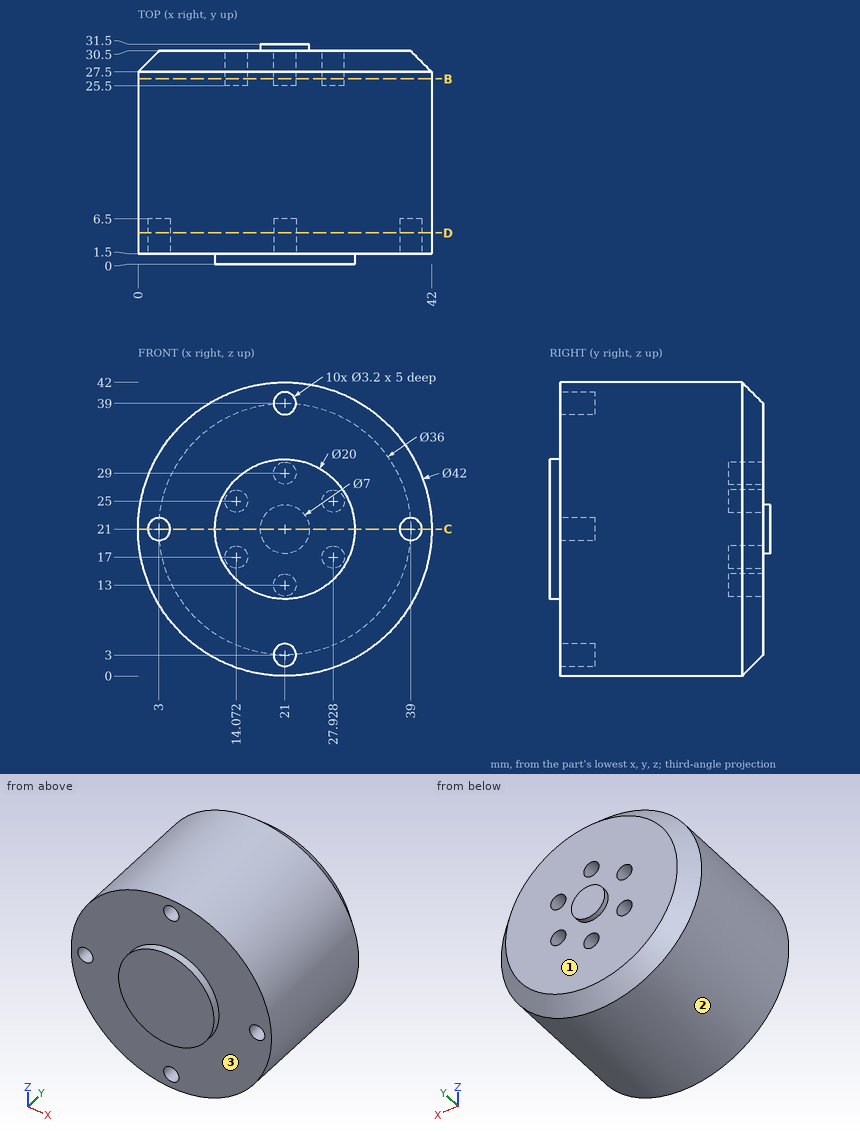
Study the drawing (mm; zero at the part's minimum x, y, z) and answer. Give positions to 0.01 mm unless a question says otherwise; leave off trailing zeros. Loops run counter-clockwise (first coordinate to the right, second up) from the corner with the lowest first, then second, coordinate; pieces in that order, holes last. Notation, with made-up numbers: M 20.25,49 L 48.25,49 A24 cw 48.25,63 Z; hole C 12.25,0 d7. An arc over 180 degrees is marked long. One line per item, written item: value.
1. Find the intervals of material crossed by probe 1 along X at (y, z) = (26, 25) (1 decimal); probe 2 along X at (y, z) = (28.3, 17); probe 3 along Z at (x, y) = (29, 27), in increasing order.
Found:
probe 1: 0.4 to 12.5, 15.7 to 26.3, 29.5 to 41.6
probe 2: 1.2 to 12.47, 15.67 to 26.33, 29.53 to 40.8
probe 3: 1.58 to 15.81, 18.19 to 23.81, 26.19 to 40.42
2. Each of these flat-tipped pins is pushed along its axis until it touches: P1, Ø12, axis at x = 13.5, y = 28, coming from the +Z side (3 decimals); P2, Ø1.6, axis at x = 28.5, z = 25, coming from the +Y side; P3, Ø1.9, axis at x = 39, z = 21, coming from the +Y side. Where does it stop, or does it pass through?
Found:
P1: z = 41.945
P2: y = 25.5
P3: y = 30.5
3. For a pull along Y with two mould halves and no side action, classify the marked faces 1, 2 and 3 as pulls with the +Y half, pulls with the -Y half, needs draft (parallel to the pull), parting line crosses it, or undercut.
Found:
face 1: pulls with the +Y half
face 2: needs draft
face 3: pulls with the -Y half
4. Section B-B on y = 26.5 is taken. Determine the outline of the cut face in (x, z), plus the area to 3 significant figures.
Found:
outline: C 21,21 d42; hole C 14.07,17 d3.2; hole C 14.07,25 d3.2; hole C 21,13 d3.2; hole C 21,29 d3.2; hole C 27.93,17 d3.2; hole C 27.93,25 d3.2
area: 1,340 mm^2
5. Section D-D on y = 4.5 is taken. Determine the outline of the cut face in (x, z), plus the area to 3 significant figures.
Found:
outline: C 21,21 d42; hole C 3,21 d3.2; hole C 21,3 d3.2; hole C 21,39 d3.2; hole C 39,21 d3.2
area: 1,350 mm^2
6. Section C-C on z = 21 is taken. Determine the outline of the cut face in (x, y).
Found:
outline: M 0,1.5 L 1.4,1.5 L 1.4,6.5 L 4.6,6.5 L 4.6,1.5 L 11,1.5 L 11,0 L 31,0 L 31,1.5 L 37.4,1.5 L 37.4,6.5 L 40.6,6.5 L 40.6,1.5 L 42,1.5 L 42,27.5 L 39,30.5 L 24.5,30.5 L 24.5,31.5 L 17.5,31.5 L 17.5,30.5 L 3,30.5 L 0,27.5 Z
